from build123d import *

# Parameters (mm, degrees)
SKETCH_2_R               = 101.541015805
CUT_EXTRUDE_1_DEPTH      = 92
SKETCH_4_R               = 60
SKETCH_4_R_2             = 39
EXTRUDE_1_DEPTH          = 1.5
SKETCH_5_W               = 2
SKETCH_5_H               = 2
SKETCH_6_R               = 3
CUT_EXTRUDE_2_DEPTH      = 20
PATTERN_CIRCULAR_1_COUNT = 8


with BuildPart() as part:
    # 草图1 → 旋转1 (revolve)
    with BuildSketch(Plane(origin=(0, 0, 0), x_dir=(0, 0, -1), z_dir=(1, 0, 0))):
        with BuildLine():
            Line((-40, 0), (40, 0))
            ThreePointArc((40, 0), (0, 40), (-40, 0))
        make_face()
    revolve(axis=Axis((0, 0, 40), (0, 0, -1)))

    # 草图2 → 切除-拉伸1 (cut)
    with BuildSketch(Plane.XY):
        with Locations((-18.762206379, 13.237665106)):
            Circle(SKETCH_2_R)
    extrude(amount=-CUT_EXTRUDE_1_DEPTH, mode=Mode.SUBTRACT)

    # 草图3 → 切除-旋转1 (revolve, cut)
    with BuildSketch(Plane(origin=(0, 0, 0), x_dir=(1, 0, 0), z_dir=(0, 1, 0))):
        with BuildLine():
            Line((0, 38.5), (0, -38.5))
            ThreePointArc((0, -38.5), (38.5, 0), (0, 38.5))
        make_face()
    revolve(axis=Axis((0, 0, -38.5), (0, 0, 1)), mode=Mode.SUBTRACT)

    # 草图4 → 凸台-拉伸1 (add)
    with BuildSketch(Plane(origin=(0, 0, 0), x_dir=(-1, 0, 0), z_dir=(0, 0, -1))):
        Circle(SKETCH_4_R)
        Circle(SKETCH_4_R_2, mode=Mode.SUBTRACT)
    extrude(amount=-EXTRUDE_1_DEPTH)

    # 草图5 → 旋转2 (revolve)
    with BuildSketch(Plane(origin=(0, 0, 0), x_dir=(1, 0, 0), z_dir=(0, 1, 0)), mode=Mode.PRIVATE) as revolve_2_sk:
        with Locations((-44, 1)):
            Rectangle(SKETCH_5_W, SKETCH_5_H)
    revolve(revolve_2_sk.sketch.rotate(Axis((0, 0, -24.660694069), (0, 0, 1)), 270), axis=Axis((0, 0, -24.660694069), (0, 0, 1)))

    # 草图6 → 切除-拉伸2 (cut)
    with BuildSketch(Plane.XY.offset(1.5)):
        with Locations((52, 0)):
            Circle(SKETCH_6_R)
    cut_extrude_2 = extrude(amount=-CUT_EXTRUDE_2_DEPTH, mode=Mode.SUBTRACT)

    # 阵列(圆周)1: 切除-拉伸2 ×8 about axis
    pattern_circular_1_axis = Axis((0, 0, 0), (0, 0, 1))
    for i in range(1, PATTERN_CIRCULAR_1_COUNT):
        add(cut_extrude_2.rotate(pattern_circular_1_axis, i * 360 / PATTERN_CIRCULAR_1_COUNT), mode=Mode.SUBTRACT)


solid = part.part
The listing builds one solid part. Answer for the finished solid, in the listing's coordinates (mm). A direction names the side the tool comes from. Round coordinates to 2 decimals unless told otherwise and drop trailing zeros. Order: outer loops, then holes, each group sorted by start corner. A loop starts at its lowest first (then second) coordinate and runs counter-clockwise, first axis right, second up. Notation, with made-up numbers: (7, 62) -> (43, 62) arc R26 cw to (43, 77) -> close; hole circle Ø3 at (26, 5.25). An arc over 180 degrees is marked (long way). Put each result on its own line as item: value.
Q1. Consider line 1 along X through (y, z) = (0, -1.5); line 2 along Z through (x, y) = (-48.5, -4); line 3 along X through (y, z) = (-52, 0.4). Determine where each line is inside the solid, lowest interval first.
Results list:
line 1: -45 to -43, 43 to 45
line 2: 0 to 1.5
line 3: -29.93 to -3, 3 to 29.93
Q2. Which of the six approach directions +Z, -Z, +X, -X, +Y, -Y give full straight-line access (tool end or side, diameter ignored) to faces 1 (the flat face through (32, -22, 0)), 2 (the cylindrical face through (0, 49, 1))?
Results list:
face 1: -Z
face 2: +Z, -Z
Q3. Section C-C, the plane x = -52 is taken. Write down the section's boundary in (y, z), and give its area (3 significant figures).
Results list:
outline: (-29.93, 0) -> (-3, 0) -> (-3, 1.5) -> (-29.93, 1.5) -> close; (3, 0) -> (29.93, 0) -> (29.93, 1.5) -> (3, 1.5) -> close
area: 80.8 mm^2
Q4. Determine the mould class of faces 3 (the flat face through (-12, -39, 1.5)), 4 (the cylindrical face through (0, -49, 1)), 5 (the cylindrical face through (59.94, 2.64, 0.74)) for opening direction Y: pulls with the +Y half, pulls with the -Y half, needs draft (parallel to the pull), parting line crosses it, or undercut.
Results list:
face 3: needs draft
face 4: undercut
face 5: parting line crosses it
Q5. Each of these flat-tipped pins is pushed along its axis until it touches: P1, Ø6, axis at x = -15.5, y = -6, coming from the -Z side; P2, Ø8, axis at x = -52, y = 0, coming from the -Z side; P3, Ø2, axis at x = 3, z = 8.5, coming from the -Y side. Where does it stop, or does it pass through?
Results list:
P1: z = 33.13
P2: z = 0
P3: y = -39.19
Q6. Section B-B, the plane y = 0 is taken. Write down the section's boundary in (x, z).
Results list:
outline: (-60, 0) -> (-55, 0) -> (-55, 1.5) -> (-60, 1.5) -> close; (-49, 0) -> (-45, 0) -> (-45, -2) -> (-43, -2) -> (-43, 0) -> (-38.5, 0) arc R38.5 cw to (38.5, 0) -> (43, 0) -> (43, -2) -> (45, -2) -> (45, 0) -> (49, 0) -> (49, 1.5) -> (39.97, 1.5) arc R40 ccw to (-39.97, 1.5) -> (-49, 1.5) -> close; (55, 0) -> (60, 0) -> (60, 1.5) -> (55, 1.5) -> close
